Verification items for the finished model (mm, model axes). A direction names the side the tool comes from. Give positions to 0.01 mm unless a question says otherwise; leave off trailing zeros. Loops run counter-clockwise (first coordinate to the right, second up) from the corner with the lowest first, then second, coordinate; pieces in that order, holes last. Notation, with made-up numbers: M -17.75,-17.75 L -7.75,-17.75 A23 cw -7.75,11.25 Z; hole C 52,-26.5 d11. An arc over 180 degrees is marked long. Use CSV: the item, a comma, the result in double quotes.
from build123d import *

# Parameters (mm, degrees)
F1_DEPTH  = 20
F2_R      = 5
F3_W      = 15.9383661317
F3_H      = 2
F4_DEPTH  = 15
F5_W      = 20
F5_H      = 12
F6_DEPTH  = 2
F7_W      = 20
F7_H      = 12
F8_DEPTH  = 15.2
F9_W      = 20
F9_H      = 12
F10_DEPTH = 25


with BuildPart() as f1:
    # F0 (on Top) → F1 (new body)
    with BuildSketch(Plane.XY):
        Polygon((20.42718686, -51.6759875909), (-29.57281314, -51.6759875909), (-29.57281314, -53.6759875909), (22.42718686, -53.6759875909), (22.42718686, 51.4633835634), (-22.8882024919, 30.3324704763), (-22.0429659684, 28.5198549023), (20.42718686, 48.3240124091), align=None)
    extrude(amount=F1_DEPTH)

    # F2
    f2_edges = [f1.edges().sort_by_distance(p)[0] for p in [
        (20.427187, 48.324012, 10),
        (20.427187, -51.675988, 10),
    ]]
    fillet(f2_edges, radius=F2_R)

    # F3 (on face) → F4 (join)
    with BuildSketch(Plane.XY.offset(20)):
        with Locations((-21.6036300742, -52.6759875909)):
            Rectangle(F3_W, F3_H)
    extrude(amount=F4_DEPTH)

    # F5 (on face) → F6 (cut, through all)
    with BuildSketch(Plane.YZ.offset(22.42718686)):
        with Locations((-33.6759875909, 10)):
            Rectangle(F5_W, F5_H)
        with Locations((-3.6759875909, 10)):
            Rectangle(F5_W, F5_H)
        with Locations((26.3240124091, 10)):
            Rectangle(F5_W, F5_H)
    extrude(amount=-F6_DEPTH, mode=Mode.SUBTRACT)

    # F7 (on face) → F8 (cut)
    with BuildSketch(Plane(origin=(-15.7059849883, 33.6815935008, 0), x_dir=(-0.906307787, -0.4226182617, 0), z_dir=(-0.4226182617, 0.906307787, 0))):
        with Locations((-17.1167086999, 10)):
            Rectangle(F7_W, F7_H)
    extrude(amount=-F8_DEPTH, mode=Mode.SUBTRACT)

    # F9 (on face) → F10 (cut)
    with BuildSketch(Plane.XZ.offset(53.6759875909)):
        with Locations((2.42718686, 10)):
            Rectangle(F9_W, F9_H)
    extrude(amount=-F10_DEPTH, mode=Mode.SUBTRACT)


solid = f1.part
(1) Section check C-C on x = -19. Record the cut outline in (y, z).
Calculated:
outline,"M -53.68,0 L -51.68,0 L -51.68,35 L -53.68,35 Z; M 29.94,0 L 32.15,0 L 32.15,20 L 29.94,20 Z"
(2) Section check A-A on y = -41. Record the cut outline in (x, z), plus the area to 3 significant figures.
Calculated:
outline,"M 20.43,0 L 22.43,0 L 22.43,4 L 20.43,4 Z; M 20.43,16 L 22.43,16 L 22.43,20 L 20.43,20 Z"
area,"16.0 mm²"
(3) Section check D-D on z = 18.5. Record the cut outline in (x, y), plus the area to 3 significant figures.
Calculated:
outline,"M -29.57,-53.68 L 22.43,-53.68 L 22.43,51.46 L -22.89,30.33 L -22.04,28.52 L 13.31,45.01 A5 cw 20.43,40.48 L 20.43,-46.68 A5 cw 15.43,-51.68 L -29.57,-51.68 Z"
area,"424 mm²"
(4) Scan lines: L1, parallel to Y at x = -23, z = 28; L2, parallel to Y at x = 7, z = 1.5; L3, parallel to Z at x = -4, y = 37.5. Record each from-to range of solid material in increasing order. Write a range as from..to.
Calculated:
L1,"y = -53.68..-51.68"
L2,"y = -53.68..-51.68, 42.06..44.27"
L3,"z = 0..4, 16..20"
(5) Section check B-B on z = 6.5. Count the separate pieces of the cut face and the enclosed holes in it, plus the area to 3 significant figures.
Calculated:
separate pieces,"6"
enclosed holes,"0"
area,"224 mm²"
(6) Depth check by flat-ended pin: pin 1 Ø10 at (x, z) = (0.5, 29.5) entering from -Y; pin 2 Ø5 at (x, y) = (1.5, 39) entering from +Z; pin 3 Ø0.6 at (x, z) = (21.5, 8.5) entering from +Y; pin 4 Ø10.5 at (x, z) = (-0.5, 24.5) entering from +Y. Enter the tip coordinate at first touch or a pass-through.
Calculated:
pin 1,"passes through"
pin 2,"stops at z = 20"
pin 3,"stops at y = 51.17"
pin 4,"stops at y = 42.03"
(7) Mould release check, pull along Y, two halves, no side actions. Record for faces 6 (the flat face through (-10, -53.676, 13)), 7 (the flat face through (21, 6.324, 10)), 8 (the flat face through (-29.573, -53, 17)): released by +Y, released by -Y, zero draft, split by the parting line, or undercut.
Calculated:
face 6,"released by -Y"
face 7,"undercut"
face 8,"zero draft"
(8) Tool access check on faces 1 (the flat face through (0.087, 41.046, 3.193)), 2 (the flat face through (12.427, -53, 10)), 3 (the flat face through (21, -13.676, 10)), 4 (the flat face through (-22, -53, 35)), 5 (the flat face through (-12.469, 32.984, 9.86)). Record the directions out of +Z, -Z, +X, -X, +Y, -Y that give a thin tool (end or side, any length) a straight path to the whole face; none if there is none.
Calculated:
face 1,"+Z, -Z, -X, +Y"
face 2,"-Y"
face 3,"+X, -X"
face 4,"+Z, +X, -X, +Y, -Y"
face 5,"+Z, -Z"
